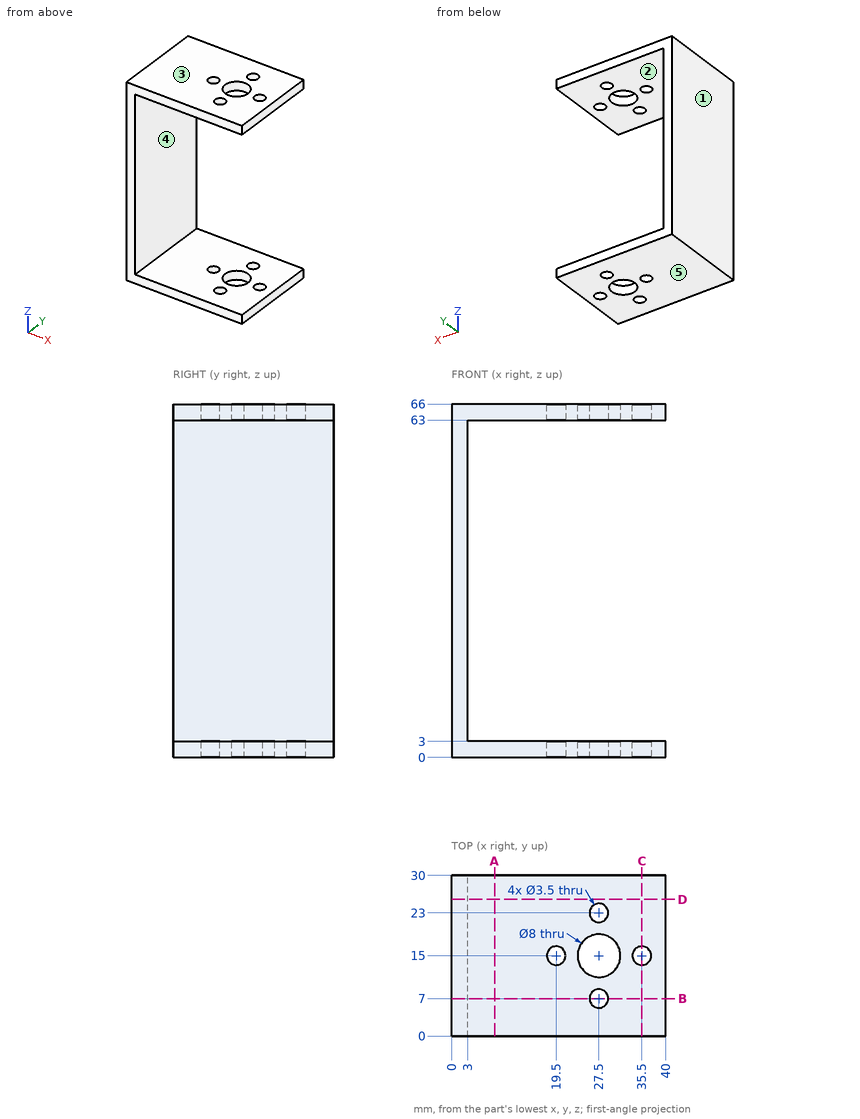
Design review of the part shown in the three views and the two pictorial views. Dimensions are in mm from the part's minimum x, y and z. A direction names the side the tool comes from. Give positions to 0.01 mm unless a question says otherwise; leave off trailing zeros. Write each loop counter-clockwise with the first axis right and the second up, starting at its lowest first coordinate (ties: lowest second). Pieces come first, ordered by that corner, then holes.
Item 1: Wall thickness on probe 1 along Y at (x, z) = (27.5, 64.85); probe 2 along Z at (x, y) = (37.5, 4.5); probe 3 along Y at (x, z) = (19.5, 1.15): over which ranges is each line inside the solid? List them lowest first.
Item 2: Take a section at A-A (x = 8). Give the boundary of the cut face in (y, z), and give its area (3 significant figures).
Item 3: Take a section at C-C (x = 35.5). Give the boundary of the cut face in (y, z), and give its area (3 significant figures).
Item 4: The part is to be moulded in two halves that separate along Z. For the marked faces 3, 4 and 5, say which applies: +Z half, -Z half, draft (parallel to the pull), parting line (faces both ways), or undercut.
Item 5: Take a section at D-D (y = 25.5). Give the boundary of the cut face in (x, z), and give its area (3 significant figures).
Item 6: Take a section at B-B (y = 7). Give the boundary of the cut face in (x, z).
Item 7: Machinability: for the marked faces 1 and 2, which of the approach directions +Z, -Z, +X, -X, +Y, -Y give a long, thin tool a straight path to every point of the face, cutting with its end or side? Answer none if there is none.
Item 8: Insertion check: P1, Ø15, axis at y = 22.5, z = 32.5, coming from the +X side. The pin has a flat end and moves straight along its axis. Give the tip position at first contact, or say it passes through.
Established:
1. probe 1: y = 0 to 5.25, 8.75 to 11, 19 to 21.25, 24.75 to 30
1. probe 2: z = 0 to 3, 63 to 66
1. probe 3: y = 0 to 13.25, 16.75 to 30
2. outline: (0, 0) - (30, 0) - (30, 3) - (0, 3) - close; (0, 63) - (30, 63) - (30, 66) - (0, 66) - close
2. area: 180 mm2
3. outline: (0, 0) - (13.25, 0) - (13.25, 3) - (0, 3) - close; (0, 63) - (13.25, 63) - (13.25, 66) - (0, 66) - close; (16.75, 0) - (30, 0) - (30, 3) - (16.75, 3) - close; (16.75, 63) - (30, 63) - (30, 66) - (16.75, 66) - close
3. area: 159 mm2
4. face 3: +Z half
4. face 4: undercut
4. face 5: -Z half
5. outline: (0, 0) - (40, 0) - (40, 3) - (3, 3) - (3, 63) - (40, 63) - (40, 66) - (0, 66) - close
5. area: 420 mm2
6. outline: (0, 0) - (25.75, 0) - (25.75, 3) - (3, 3) - (3, 63) - (25.75, 63) - (25.75, 66) - (0, 66) - close; (29.25, 0) - (40, 0) - (40, 3) - (29.25, 3) - close; (29.25, 63) - (40, 63) - (40, 66) - (29.25, 66) - close
7. face 1: +Z, -Z, -X, +Y, -Y
7. face 2: +X, +Y, -Y
8. P1: stops at x = 3
